Source: CAD feature listing. Evaluate the final solid. Frame: model axes, mm. Round coordinates to 2 decimals unless told otherwise and drop trailing zeros. Write each loop counter-clockwise with the first axis right and the second up, starting at its lowest first coordinate (ties: lowest second). Pieces come first, ordered by that corner, then holes.
from build123d import *

# Parameters (mm, degrees)
F0_R            = 41.5
F1_DEPTH        = 6
F2_W            = 150
F2_H            = 150
F3_DEPTH        = 6
F5_R            = 17.5
F6_DEPTH        = 6.001
F7_D            = 12.6
F7_COPIES_COUNT = 6
F9_D            = 9.8044


# Not quite as in the source:
# - a pattern or mirror of a feature is missing from the dataset's text; its kind, count and spacing are read off the source's solid


with BuildPart() as f1:
    # F0 (on Top) → F1 (new body)
    with BuildSketch(Plane.XY):
        Circle(F0_R)
    extrude(amount=F1_DEPTH)

    # F2 (on Top) → F3 (join)
    with BuildSketch(Plane.XY):
        Rectangle(F2_W, F2_H)
    extrude(amount=F3_DEPTH)

    # F5 (on face) → F6 (cut, through all)
    with BuildSketch(Plane.XY.offset(6)):
        Circle(F5_R)
    extrude(amount=-F6_DEPTH, mode=Mode.SUBTRACT)

    # F7 (through all)
    with Locations(Plane.XY.offset(6)):
        with Locations((0, 32.5)):
            f7 = Hole(F7_D / 2)

    # F7_copies: F7 ×6 about axis
    f7_copies_axis = Axis((0, 0, 0), (0, 0, 1))
    for i in range(1, F7_COPIES_COUNT):
        add(f7.rotate(f7_copies_axis, i * 360 / F7_COPIES_COUNT), mode=Mode.SUBTRACT)

    # F9 (through all)
    with Locations(Plane.XY.offset(6)):
        with Locations((-50, 50), (50, 50), (50, -50), (-50, -50)):
            Hole(F9_D / 2)


solid = f1.part
1) Section query B-B on x = 50. Return the cut outline in (y, z).
Taken from the geometry:
outline: (-75, 0) - (-54.9, 0) - (-54.9, 6) - (-75, 6) - close; (-45.1, 0) - (45.1, 0) - (45.1, 6) - (-45.1, 6) - close; (54.9, 0) - (75, 0) - (75, 6) - (54.9, 6) - close
2) Section query C-C on y = 0. Return the cut outline in (x, z).
Taken from the geometry:
outline: (-75, 0) - (-17.5, 0) - (-17.5, 6) - (-75, 6) - close; (17.5, 0) - (75, 0) - (75, 6) - (17.5, 6) - close
3) Section query A-A on x = 0. Return the cut outline in (y, z).
Taken from the geometry:
outline: (-75, 0) - (-38.8, 0) - (-38.8, 6) - (-75, 6) - close; (-26.2, 0) - (-17.5, 0) - (-17.5, 6) - (-26.2, 6) - close; (17.5, 0) - (26.2, 0) - (26.2, 6) - (17.5, 6) - close; (38.8, 0) - (75, 0) - (75, 6) - (38.8, 6) - close
4) Material intervals for line 1 (Y direction, x = 50, z = 1.8); line 2 (Y direction, x = -45.5, z = 0.85); line 3 (X direction, y = 1, z = 4.5), sorted ascending.
Taken from the geometry:
line 1: y = -75 to -54.9, -45.1 to 45.1, 54.9 to 75
line 2: y = -75 to -51.94, -48.06 to 48.06, 51.94 to 75
line 3: x = -75 to -17.47, 17.47 to 75
5) Section query D-D on z = 3.55. State how many separate pieces and enclosed holes the cut face has, then the cut area to 3 significant figures.
Taken from the geometry:
separate pieces: 1
enclosed holes: 11
area: 20,500 mm2
6) Contact query for a flat-ended pin moving along its axis: P1, Ø10, axis at x = 28.15, y = 16.25, coming from the +Z side. Output: stop coordinate, or through.
Taken from the geometry:
P1: passes through
7) Pull-direction query (Y, two-part tool) for faces 1 (the face through (-18, 1, 6)), 2 (the face through (-33.965, -18.663, 2.958)), 3 (the face through (51.063, -54.786, 2.958)), 4 (the face through (-1, -75, 3)); classes: released by +Y, released by -Y, zero draft, split by the parting line, or undercut.
Taken from the geometry:
face 1: zero draft
face 2: undercut
face 3: undercut
face 4: released by -Y
